from build123d import *

# Parameters (mm, degrees)
F0_R          = 12.55
F0_R_2        = 10.9
F0_R_3        = 2.75
F0_R_4        = 5.1
F1_DEPTH      = 13.25
F2_R          = 10
F3_R          = 5
F4_R          = 3
F5_DEPTH      = 14.5510001
F5_DEPTH_BACK = 40.0072913958
F4_R_2        = 5
F6_DEPTH      = 12.5
F6_DEPTH_BACK = 40.0072913958


with BuildPart() as f1:
    # F0 (on Right) → F1 (new body, symmetric)
    with BuildSketch(Plane.YZ):
        with BuildLine():
            Line((7.45, 25.2829590551), (-23.7829060836, 25.2829590551))
            ThreePointArc((-23.7829060836, 25.2829590551), (-39.2686382031, 4.2232189691), (-14.55, -4.280278967))
            Line((-14.55, -4.280278967), (-14.55, -14.55))
            Line((-14.55, -14.55), (14.55, -14.55))
            Line((14.55, -14.55), (14.55, 18.1829590551))
            ThreePointArc((14.55, 18.1829590551), (12.4704581464, 23.2034172015), (7.45, 25.2829590551))
        make_face()
        Circle(F0_R, mode=Mode.SUBTRACT)
        with Locations((-23.7829060836, 9.059573843)):
            Circle(F0_R_2, mode=Mode.SUBTRACT)
        with Locations((-7.9205860656, 17.9829590551)):
            Circle(F0_R_3, mode=Mode.SUBTRACT)
        with Locations((7.45, 18.1829590551)):
            Circle(F0_R_4, mode=Mode.SUBTRACT)
    extrude(amount=F1_DEPTH, both=True)

    # F2
    f2_edges = [f1.edges().sort_by_distance(p)[0] for p in [
        (0, -23.782906, 25.282959),
        (0, 14.55, 18.182959),
        (0, 7.45, 25.282959),
        (0, -14.55, -14.55),
        (0, 14.55, -14.55),
    ]]
    fillet(f2_edges, radius=F2_R)

    # F3
    f3_edges = [f1.edges().sort_by_distance(p)[0] for p in [
        (0, -14.55, -4.280279),
    ]]
    fillet(f3_edges, radius=F3_R)

    # F4 (on Front) → F5 (cut, two sides)
    with BuildSketch(Plane.XZ) as f5_sk:
        with Locations((0, 5.45)):
            Circle(F4_R)
    extrude(amount=-F5_DEPTH, mode=Mode.SUBTRACT)
    extrude(f5_sk.sketch, amount=F5_DEPTH_BACK, mode=Mode.SUBTRACT)

    # F4 (on Front) → F6 (cut, two sides)
    with BuildSketch(Plane.XZ) as f6_sk:
        with Locations((0, 5.45)):
            Circle(F4_R_2)
        with Locations((0, 5.45)):
            Circle(F4_R, mode=Mode.SUBTRACT)
    extrude(amount=-F6_DEPTH, mode=Mode.SUBTRACT)
    extrude(f6_sk.sketch, amount=F6_DEPTH_BACK, mode=Mode.SUBTRACT)

    # F7 (on Right) → F8 (revolve, cut)
    with BuildSketch(Plane.YZ):
        Polygon((14.55, 5.45), (14.55, 8.45), (14.25, 8.45), (12.55, 10.45), (11.55, 10.45), (11.55, 5.45), align=None)
    revolve(axis=Axis((0, 7.275, 5.45), (0, 1, 0)), mode=Mode.SUBTRACT)


solid = f1.part
For this review, take the finished solid that the model builds, in its own axes (mm). A direction names the side the tool comes from. Give positions to 0.01 mm unless a question says otherwise; leave off trailing zeros. Order: outer loops, then holes, each group sorted by start corner. A loop starts at its lowest first (then second) coordinate and runs counter-clockwise, first axis right, second up. Notation, with made-up numbers: (-32, 24.25) - (-3, 24.25) arc R22 cw to (-3, 58.25) - close; hole circle Ø5 at (15.5, 88). An arc over 180 degrees is marked (long way). Answer as a JSON object with one key per item and string values. Group by question number.
Item 1: Take a section at C-C on z = 16.5. Give the boundary of the cut face in (x, y), and give its area (3 significant figures).
Item 2: Take a section at A-A on y = 0. Give the boundary of the cut face in (x, z).
Item 3: Clearance check with flat-ended pins moving along their axes: pin 1 Ø1 at (x, z) = (-7.5, -2.5) entering from -Y; pin 2 Ø5 at (x, z) = (6, 4) entering from -Y. State where each tip first meets the part, or that it passes through.
Item 4: Machinability: for faces 4 (the cylindrical face through (-0.19, -2.72, -12.25)), 5 (the cylindrical face through (-0.796, -12, 10.386)), which of the approach directions +Z, -Z, +X, -X, +Y, -Y give a long, thin tool a straight path to every point of the face, cutting with its end or side? Answer none if there is none.
Item 5: Take a section at B-B on y = -6. Give the boundary of the cut face in (x, z).
Item 6: Wall thickness on line 1 along Z through (x, y) = (-9, 0); line 2 along Y through (x, z) = (-11.5, 10); line 3 along Z through (x, y) = (0, 10.55): over which ranges is each line inside the solid? List them lowest first.
Item 7: Draft analysis for pull direction Y (two halves, no side actions). For faces 1 (the flat face through (0, 0, -14.55)), 2 (the cylindrical face through (-0.19, 11.7, -11.54)), 3 (the cylindrical face through (-0.19, -6.44, 20.3)), state which applies: pulls with the +Y half, pulls with the -Y half, needs draft (parallel to the pull), parting line crosses it, or undercut.
Item 8: Take a section at D-D on z = -3. Give the boundary of the cut face in (x, y), and give its area (3 significant figures).
Reported:
{
 "1": {"outline": "(-13.25, -38.2) - (13.25, -38.2) - (13.25, -31.75) - (-13.25, -31.75) - close; (-13.25, -15.82) - (13.25, -15.82) - (13.25, -10.24) - (-13.25, -10.24) - close; (-13.25, -5.6) - (13.25, -5.6) - (13.25, 2.64) - (-13.25, 2.64) - close; (-13.25, 12.26) - (13.25, 12.26) - (13.25, 14.55) - (-13.25, 14.55) - close", "area": "598 mm^2"},
 "2": {"outline": "(-13.25, -14.55) - (13.25, -14.55) - (13.25, -12.55) - (-13.25, -12.55) - close; (-13.25, 12.55) - (13.25, 12.55) - (13.25, 25.28) - (-13.25, 25.28) - close"},
 "3": {"pin 1": "y = -35.65", "pin 2": "y = -39.8"},
 "4": {"face 4": "+X, -X", "face 5": "-Y"},
 "5": {"outline": "(-13.25, -14.44) - (13.25, -14.44) - (13.25, -11.02) - (-13.25, -11.02) - close; (-13.25, 11.02) - (13.25, 11.02) - (13.25, 16.01) - (-13.25, 16.01) - close; (-13.25, 19.95) - (13.25, 19.95) - (13.25, 25.28) - (-13.25, 25.28) - close"},
 "6": {"line 1": "-14.55 to -12.55, 12.55 to 25.28", "line 2": "-39.98 to -34.64, -12.92 to -7.58, 7.58 to 14.55", "line 3": "-12.55 to -6.8, 10.45 to 14.13, 22.23 to 24.57"},
 "7": {"face 1": "needs draft", "face 2": "pulls with the +Y half", "face 3": "undercut"},
 "8": {"outline": "(-13.25, -34.63) - (13.25, -34.63) - (13.25, -12.19) - (-13.25, -12.19) - close; (-13.25, 12.19) - (13.25, 12.19) - (13.25, 14.55) - (-13.25, 14.55) - close", "area": "658 mm^2"}
}
